Autodesk Inventor part; units mm, degrees
ref_plane "rr_XY" through (-0.5, 0, 0) normal (1, 0, 0) x (0, 0, -1)
ref_plane "rr_YZ" through (-0.5, 0, 0) normal (0, 0, -1) x (0, 1, 0)
ref_plane "rr_ZX" through (-0.5, 0, 0) normal (0, 1, 0) x (1, 0, 0)
sketch "Sketch_3" plane through (0, 0, 0) normal (1, 0, 0) x (0, 1, 0)
  arc A0 (-8.5493, -5.1875) -> (-8.5493, 5.1875) centre (0, 0) ccw
  arc A1 (-8.5493, 5.1875) -> (-7.4165, 2.2351) centre (-6.8394, 4.15) ccw
  arc A2 (-7.4165, 2.2351) -> (-4.975, 4.874) centre (-6.8394, 4.15) ccw
  arc A3 (-3.9223, 7.4259) -> (-4.975, 4.874) centre (-3.1107, 5.5979) ccw
  arc A4 (-3.9223, -7.4259) -> (-3.9223, 7.4259) centre (-0.625, 0) ccw
  arc A5 (-4.975, -4.874) -> (-3.9223, -7.4259) centre (-3.1107, -5.5979) ccw
  arc A6 (-4.975, -4.874) -> (-7.4165, -2.2351) centre (-6.8394, -4.15) ccw
  arc A7 (-7.4165, -2.2351) -> (-8.5493, -5.1875) centre (-6.8394, -4.15) ccw
  circle A8 centre (-6.8394, -4.15) radius 1
  circle A9 centre (-6.8394, 4.15) radius 1
extrude "Extrusion1" add sketch "Sketch_3" along normal mid plane 1
ref_plane "rr_XY" through (-0.5, 0, 0) normal (1, 0, 0) x (0, 0, -1)
ref_plane "rr_YZ" through (-0.5, 0, 0) normal (0, 0, -1) x (0, 1, 0)
ref_plane "rr_ZX" through (-0.5, 0, 0) normal (0, 1, 0) x (1, 0, 0)
properties part number "RRING-C-INT-S-19"
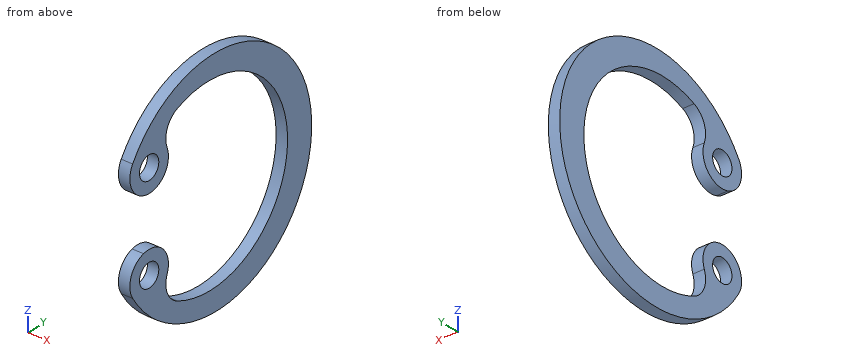
Work out the finished part from the listing and answer in its coordinate system (mm). Give positions to 0.01 mm unless a question says otherwise; leave off trailing zeros. Loops run counter-clockwise (first coordinate to the right, second up) from the corner with the lowest first, then second, coordinate; pieces in that order, holes last. Notation, with made-up numbers: (53, 25.5) - (71, 25.5) arc R8 ccw to (71, 33.5) - close; hole circle Ø7 at (-7.5, 17.25). An arc over 180 degrees is marked (long way). Answer in a Markdown table with one row per item. Add a question column.
Q1. This flat-tipped pin is pushed along its axis until it touches: P1, Ø3, axis at y = -6.84, z = 4.15, coming from the +X side. Where does it stop, or does it pass through?
Q2. The part is cut by section A-A (y = 5.25). Determine the outline of the cut face in (x, z).
Q3. The part is cut by section C-C (y = -7). Determine the outline of the cut face in (x, z), and give its area (3 significant figures).
Q4. The part is cut by section D-D (x = 0.2). State how many separate pieces and enclosed holes the cut face has, and give its area (3 significant figures).
Q5. The part is cut by section B-B (z = 4.15). Determine the outline of the cut face in (x, y).
Q6. Consider line 1 along Z through (x, y) = (-0.4, -6); line 2 along Y through (x, z) = (-0.25, -5); line 3 along Z through (x, y) = (-0.1, -2.25). Determine where each line is inside the solid, lowest interval first.
Solution:
| question | item | result |
|---|---|---|
| 1 | P1 | stops at x = 0.5 |
| 2 | outline | (-0.5, -8.51) - (0.5, -8.51) - (0.5, -5.61) - (-0.5, -5.61) - close; (-0.5, 5.61) - (0.5, 5.61) - (0.5, 8.51) - (-0.5, 8.51) - close |
| 3 | outline | (-0.5, -7.14) - (0.5, -7.14) - (0.5, -5.14) - (-0.5, -5.14) - close; (-0.5, -3.16) - (0.5, -3.16) - (0.5, -2.16) - (-0.5, -2.16) - close; (-0.5, 2.16) - (0.5, 2.16) - (0.5, 3.16) - (-0.5, 3.16) - close; (-0.5, 5.14) - (0.5, 5.14) - (0.5, 7.14) - (-0.5, 7.14) - close |
| 3 | area | 6.02 mm² |
| 4 | separate pieces | 1 |
| 4 | enclosed holes | 2 |
| 4 | area | 110 mm² |
| 5 | outline | (-0.5, -8.84) - (0.5, -8.84) - (0.5, -7.84) - (-0.5, -7.84) - close; (-0.5, -5.84) - (0.5, -5.84) - (0.5, -4.84) - (-0.5, -4.84) - close; (-0.5, 6.36) - (0.5, 6.36) - (0.5, 9.1) - (-0.5, 9.1) - close |
| 6 | line 1 | z = -8 to -4.69, -3.61 to -2.33, 2.33 to 3.61, 4.69 to 8 |
| 6 | line 2 | y = -8.65 to -7.37, -6.31 to -5.02, 5.78 to 8.66 |
| 6 | line 3 | z = -9.74 to -7.96, 7.96 to 9.74 |
